```python
from build123d import *

# Parameters (mm, degrees)
SKETCH1_W           = 34.13125
SKETCH1_H           = 22.0265625
BOSS_EXTRUDE1_DEPTH = 1.651
FILLET1_R           = 2.54
SKETCH2_R           = 1.64
CUT_EXTRUDE1_DEPTH  = 2.54


with BuildPart() as part:
    # Sketch1 → Boss-Extrude1 (new body)
    with BuildSketch(Plane(origin=(0, 0, 0), x_dir=(1, 0, 0), z_dir=(0, 1, 0))):
        with Locations((17.065625, 11.01328125)):
            Rectangle(SKETCH1_W, SKETCH1_H)
    extrude(amount=BOSS_EXTRUDE1_DEPTH)

    # Fillet1
    fillet1_edges = [part.edges().sort_by_distance(p)[0] for p in [
        (0, 0.8255, -22.0265625),
        (34.13125, 0.8255, -22.0265625),
        (34.13125, 0.8255, 0),
        (0, 0.8255, 0),
    ]]
    fillet(fillet1_edges, radius=FILLET1_R)

    # Sketch2 → Cut-Extrude1 (cut)
    with BuildSketch(Plane(origin=(0, 1.651, 0), x_dir=(1, 0, 0), z_dir=(0, 1, 0))):
        with Locations(Location((22.92125, 18.5865625, 0), (0, 0, 270))):
            Circle(SKETCH2_R)
        with Locations(Location((22.92125, 3.44, 0), (0, 0, 270))):
            Circle(SKETCH2_R)
    extrude(amount=-CUT_EXTRUDE1_DEPTH, mode=Mode.SUBTRACT)


solid = part.part
```
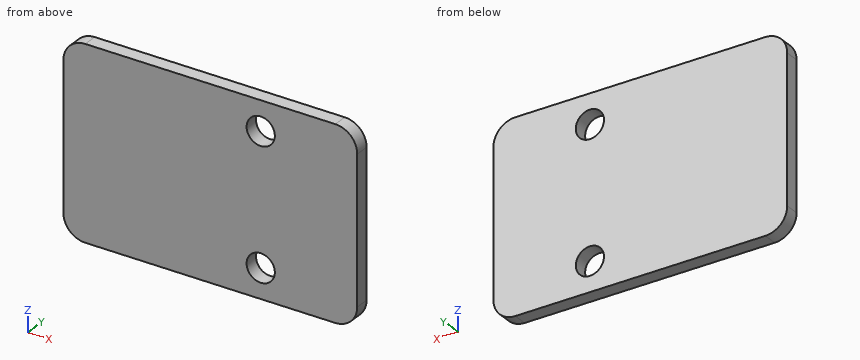
Work out the finished part from the listing and answer in its coordinate system (mm). Give positions to 0.01 mm unless a question says otherwise; leave off trailing zeros. Loops run counter-clockwise (first coordinate to the right, second up) from the corner with the lowest first, then second, coordinate; pieces in that order, holes last. Notation, with made-up numbers: (63, 34.25) -> (98, 34.25) arc R12 ccw to (98, 55.25) -> close; hole circle Ø2 at (37, 81.25). An arc over 180 degrees is marked (long way). Put each result on its own line as item: value. Start each with the question number.
Item 1: The part is cut by section A-A (z = -3.44). Give the vertices of the cut face in (x, y).
Item 2: Find the intervals of material crossed by L1, parallel to X at y = 0.5, z = -3.44; L2, parallel to Z at x = 24, y = 0.85; L3, parallel to X at y = 1.5, z = -20, in increasing order. Write a range as [from, to].
Item 3: This flat-tipped pin is pushed along its axis until it touches: P1, Ø2, axis at x = 22.92, z = -3.44, coming from the +Y side. Where does it stop, or does it pass through?
Item 4: The part is cut by section B-B (y = 0.3). Give the vertices of the cut face in (x, z).
Answers below:
1. outline: (0, 0) -> (21.28, 0) -> (21.28, 1.65) -> (0, 1.65) -> close; (24.56, 0) -> (34.13, 0) -> (34.13, 1.65) -> (24.56, 1.65) -> close
2. L1: [0, 21.28], [24.56, 34.13]
2. L2: [-22.03, -19.82], [-17.35, -4.68], [-2.2, 0]
2. L3: [0.05, 22.09], [23.75, 34.08]
3. P1: through
4. outline: (0, -19.49) arc R2.54 ccw to (2.54, -22.03) -> (31.59, -22.03) arc R2.54 ccw to (34.13, -19.49) -> (34.13, -2.54) arc R2.54 ccw to (31.59, 0) -> (2.54, 0) arc R2.54 ccw to (0, -2.54) -> close; hole circle Ø3.28 at (22.92, -18.59); hole circle Ø3.28 at (22.92, -3.44)
